Here's the drawing with two shaded views (mm, measured from the low corner). I have some questions. A direction names the side the tool comes from. Round coordinates to 2 decimals unless told otherwise and drop trailing zeros. Loops run counter-clockwise (first coordinate to the right, second up) from the corner with the lowest first, then second, coordinate; pieces in that order, holes last.
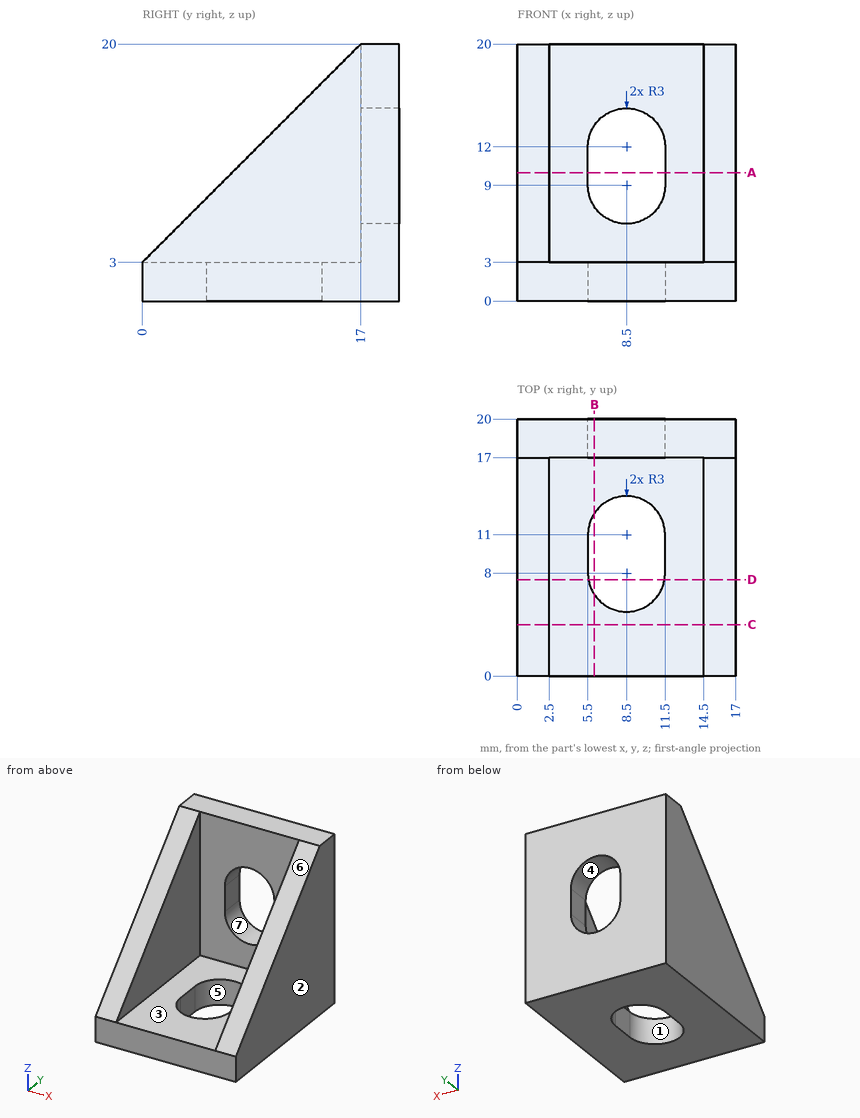
(1) If we section it at C-C, the plane y = 4: List the corners of the cut face in (x, z) for me, then the cut area to 3 significant figures.
Worked answers:
outline: (0, 0) - (17, 0) - (17, 7) - (14.5, 7) - (14.5, 3) - (2.5, 3) - (2.5, 7) - (0, 7) - close
area: 71.0 mm2
(2) For the marked faces 1, 2 and 3, which set-ups out of +Z, -Z, +X, -X, +Y, -Y let a thin tool reach every point of the face, with its end or its side?
Worked answers:
face 1: +Z, -Z
face 2: +Z, -Z, +X, +Y, -Y
face 3: +Z, -Y
(3) If we mould it in two halves opening along Z, with no side actions, what happens to the marked faces 4, 5, 6 and 7? For each: released by +Z, released by -Z, zero draft, split by the parting line, or undercut.
Worked answers:
face 4: undercut
face 5: zero draft
face 6: released by +Z
face 7: undercut
(4) If I drill on line 1 (X direction, y = 4.75, z = 6.25); line 2 (X direction, y = 17.25, z = 10.25); line 3 (Z direction, x = 6.5, y = 15.5), over which ranges is the centre line in solid material (lowest first)?
Worked answers:
line 1: x = 0 to 2.5, 14.5 to 17
line 2: x = 0 to 5.5, 11.5 to 17
line 3: z = 0 to 3
(5) Will these pins go through, and if not, where does the flat tip stop? P1, Ø4, axis at y = 10, z = 16, coming from the +X side; P2, Ø4, axis at x = 12, y = 14, coming from the +Z side.
Worked answers:
P1: passes through
P2: stops at z = 3
(6) If we section it at A-A, the plane z = 10: List the corners of the cut face in (x, y) for me.
Worked answers:
outline: (0, 7) - (2.5, 7) - (2.5, 17) - (5.5, 17) - (5.5, 20) - (0, 20) - close; (11.5, 17) - (14.5, 17) - (14.5, 7) - (17, 7) - (17, 20) - (11.5, 20) - close
(7) If we section it at B-B, the plane x = 6: List the corners of the cut face in (y, z) for me, then the cut area to 3 significant figures.
Worked answers:
outline: (0, 0) - (6.34, 0) - (6.34, 3) - (0, 3) - close; (12.66, 0) - (20, 0) - (20, 7.34) - (17, 7.34) - (17, 3) - (12.66, 3) - close; (17, 13.66) - (20, 13.66) - (20, 20) - (17, 20) - close
area: 73.1 mm2
(8) If we section it at D-D, the plane y = 7.5: List the corners of the cut face in (x, z) for me.
Worked answers:
outline: (0, 0) - (5.54, 0) - (5.54, 3) - (2.5, 3) - (2.5, 10.5) - (0, 10.5) - close; (11.46, 0) - (17, 0) - (17, 10.5) - (14.5, 10.5) - (14.5, 3) - (11.46, 3) - close
